Read the model definition and answer for the solid it produces. Units are mm, in the model's axes. Face numbers are marked on the shaded views. A direction names the side the tool comes from. Coordinates: 2 decimals unless noted, no trailing zeros. Loops run counter-clockwise (first coordinate to the right, second up) from the corner with the lowest first, then second, coordinate; pieces in that order, holes last.
from build123d import *

# Parameters (mm, degrees)
F0_W     = 90.0560617447
F0_H     = 106.9972887635
F0_W_2   = 66.873319447
F0_H_2   = 90.0560542941
F1_DEPTH = 56.642
F2_W     = 16.9049244328
F2_H     = 51.2000992894
F3_DEPTH = 25.4
F4_W     = 15.7775770826
F4_H     = 56.1789758503
F5_DEPTH = 25.4
F6_R     = 10.5970708349
F7_DEPTH = 25.4
F8_R     = 12.3308316968
F9_DEPTH = 25.4


with BuildPart() as f1:
    # F0 (on Right) → F1 (new body)
    with BuildSketch(Plane.YZ):
        Rectangle(F0_W, F0_H)
        Rectangle(F0_W_2, F0_H_2, mode=Mode.SUBTRACT)
    extrude(amount=F1_DEPTH)

    # F2 (on face) → F3 (cut)
    with BuildSketch(Plane(origin=(0, 45.0280308723, 0), x_dir=(-1, 0, 0), z_dir=(0, 1, 0))):
        with Locations((-48.1895377836, 0)):
            Rectangle(F2_W, F2_H)
    extrude(amount=-F3_DEPTH, mode=Mode.SUBTRACT)

    # F4 (on face) → F5 (cut)
    with BuildSketch(Plane.XZ.offset(45.0280308723)):
        with Locations((48.7532114587, 0)):
            Rectangle(F4_W, F4_H)
    extrude(amount=-F5_DEPTH, mode=Mode.SUBTRACT)

    # F6 (on face) → F7 (cut)
    with BuildSketch(Plane.XY.offset(53.4986443818)):
        with Locations((30.5786505342, 0)):
            Circle(F6_R)
    extrude(amount=-F7_DEPTH, mode=Mode.SUBTRACT)

    # F8 (on face) → F9 (cut)
    with BuildSketch(Plane(origin=(0, 0, -53.4986443818), x_dir=(1, 0, 0), z_dir=(0, 0, -1))):
        with Locations((34.0463332832, 0)):
            Circle(F8_R)
    extrude(amount=-F9_DEPTH, mode=Mode.SUBTRACT)


solid = f1.part
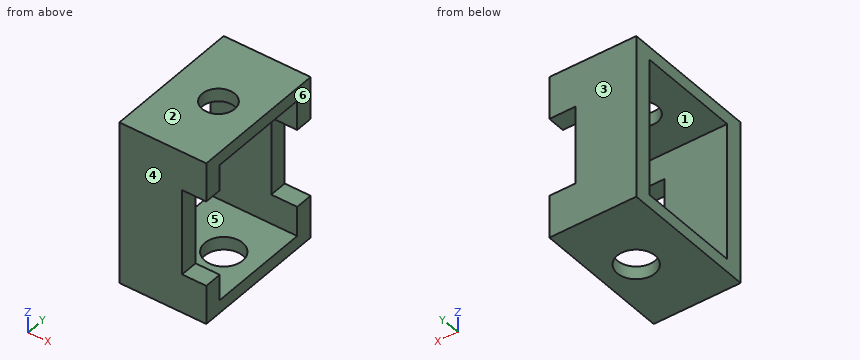
Q1. A cutting plane is placed at B-B (y = 14). Give the vertices of the cut face in (x, z), then the cut area to 3 significant figures.
Findings below:
outline: (0, -53.5) - (56.64, -53.5) - (56.64, -45.03) - (0, -45.03) - close; (0, 45.03) - (56.64, 45.03) - (56.64, 53.5) - (0, 53.5) - close
area: 960 mm2
Q2. Straight lines are drawn through the part: probe 1 along Z at (x, y) = (46.5, -19.5); probe 2 along Y at (x, z) = (18.5, 26); probe 3 along Z at (x, y) = (52, 34.5). For each, find the intervals that lie inside material, in ascending order.
Findings below:
probe 1: z = -53.5 to -45.03, 45.03 to 53.5
probe 2: y = -45.03 to -33.44, 33.44 to 45.03
probe 3: z = -53.5 to -25.6, 25.6 to 53.5
Q3. Determine the mould class of the marked faces 1, 2, 3 and 4 for opening direction Y: +Y half, -Y half, draft (parallel to the pull), parting line (faces both ways), or undercut.
Findings below:
face 1: undercut
face 2: draft
face 3: +Y half
face 4: -Y half
Q4. A cutting plane is placed at A-A (z = -4). Give the vertices of the cut face in (x, y), then the cut area to 3 significant figures.
Findings below:
outline: (0, -45.03) - (40.86, -45.03) - (40.86, -33.44) - (0, -33.44) - close; (0, 33.44) - (39.74, 33.44) - (39.74, 45.03) - (0, 45.03) - close
area: 934 mm2
Q5. Which of the six approach directions +Z, -Z, +X, -X, +Y, -Y give full straight-line access (tool end or side, diameter ignored) to the marked faces 5 and 6?
Findings below:
face 5: +X, -X
face 6: +Z, -Z, +X, +Y, -Y
Q6. A cutting plane is placed at C-C (x = 49.5). Give the vertices of the cut face in (y, z), then the cut area to 3 significant figures.
Findings below:
outline: (-45.03, -53.5) - (45.03, -53.5) - (45.03, -25.6) - (33.44, -25.6) - (33.44, -45.03) - (-33.44, -45.03) - (-33.44, -28.09) - (-45.03, -28.09) - close; (-45.03, 28.09) - (-33.44, 28.09) - (-33.44, 45.03) - (33.44, 45.03) - (33.44, 25.6) - (45.03, 25.6) - (45.03, 53.5) - (-45.03, 53.5) - close
area: 2,370 mm2
Q7. Flat-ended cylindrical pins translate along their axes: pin 1 Ø13 at (y, z) = (-41.5, -9.5) entering from +X; pin 2 Ø9.5 at (y, z) = (38, 4.5) entering from +X. Find the tip coordinate at first contact, or state that the pin passes through.
Findings below:
pin 1: stops at x = 40.86
pin 2: stops at x = 39.74
Q8. A cutting plane is placed at D-D (y = 0). Give the vertices of the cut face in (x, z), then the cut area to 3 significant figures.
Findings below:
outline: (0, -53.5) - (21.72, -53.5) - (21.72, -45.03) - (0, -45.03) - close; (0, 45.03) - (19.98, 45.03) - (19.98, 53.5) - (0, 53.5) - close; (41.18, 45.03) - (56.64, 45.03) - (56.64, 53.5) - (41.18, 53.5) - close; (46.38, -53.5) - (56.64, -53.5) - (56.64, -45.03) - (46.38, -45.03) - close
area: 571 mm2
